Here's how the part is built. I have some questions about the finished solid (model axes, mm). Face numbers are marked on the shaded views. Round coordinates to 2 decimals unless told otherwise and drop trailing zeros. Order: outer loops, then holes, each group sorted by start corner. A loop starts at its lowest first (then second) coordinate and runs counter-clockwise, first axis right, second up. Notation, with made-up numbers: M -20,53.25 L -15,53.25 A10 ccw -15,62.25 Z; hole C 38.25,-33.5 d7. An arc over 180 degrees is marked long. Write item = value, one per line. Start each with the question number.
Item 1: I want a section at B-B, the plane x = 45.5. List the corners of the cut face in (y, z) for me.
Item 2: I want a section at D-D, the plane x = -44. List the corners of the cut face in (y, z) for me, plus the area to 3 significant figures.
Item 3: I want a section at C-C, the plane z = 1.5. List the corners of the cut face in (x, y) for me, plus the area to 3 significant figures.
Item 4: Please list where these lines run through material, in increasing order: L1, parallel to Z at x = 26.5, y = 3.75; L2, parallel to X at y = 3.5, z = -37.5; L3, parallel to X at y = 7, z = 4.
Item 5: We'd pull the mould along X, two halves only. Please class the marked faces 1, 2, 3 and 4: pulls with the +X half, pulls with the -X half, needs draft (parallel to the pull), parting line crosses it, or undercut.
Item 6: I want a section at A-A, the plane y = 7. List the corners of the cut face in (x, z) for me, plus the area to 3 significant figures.
Item 7: I'm going to push flat-ended pins straight in: P1, Ø2.5, axis at x = -32.5, y = 6.5, coming from the -Z side; P2, Ø5, axis at x = -43.5, y = 3, coming from the -Z side; P3, Ø2.5, axis at y = 3, z = -47, coming from the +X side; P4, Ø5, axis at y = 8, z = -39.5, coming from the +X side. Where does each tip first touch, or does it pass through?
```python
from build123d import *

# Parameters (mm, degrees)
SKETCH_1_W      = 99
SKETCH_1_H      = 1.099776848
SKETCH_1_W_2    = 4.3
SKETCH_1_H_2    = 20
SKETCH_1_W_3    = 19.968743504
SKETCH_1_H_3    = 0.87958721
EXTRUDE_6_DEPTH = 10
SKETCH_1_15_W   = 99
SKETCH_1_15_H   = 18.900223152
EXTRUDE_7_DEPTH = 5


with BuildPart() as part:
    # Sketch 1 → Extrude 6 (new body)
    with BuildSketch(Plane(origin=(0, 0, 0), x_dir=(1, 0, 0), z_dir=(0, 1, 0))):
        Polygon((-63.8, 10), (-63.8, -10), (-59.5, -10), (-59.5, -8.900223152), (-59.5, 10), align=None)
        with Locations((-10, -9.450111576)):
            Rectangle(SKETCH_1_W, SKETCH_1_H)
        with Locations((61.65, 0)):
            Rectangle(SKETCH_1_W_2, SKETCH_1_H_2)
        with Locations((49.484371752, 75.060206395)):
            Rectangle(SKETCH_1_W_3, SKETCH_1_H_3)
    extrude(amount=EXTRUDE_6_DEPTH)

    # Sketch 1_15 → Extrude 7 (add)
    with BuildSketch(Plane(origin=(0, 0, 0), x_dir=(1, 0, 0), z_dir=(0, 1, 0))):
        with Locations((-10, 0.549888424)):
            Rectangle(SKETCH_1_15_W, SKETCH_1_15_H)
        Polygon((39.5, -8.900223152), (39.5, -10), (59.5, -10), (59.5, 10), (39.5, 10), align=None)
        Polygon((39.5, 74.62041279), (39.5, 10), (59.5, 10), (59.5, 75.5), (59.468743504, 75.5), (59.468743504, 74.62041279), align=None)
    extrude(amount=EXTRUDE_7_DEPTH)


solid = part.part
```
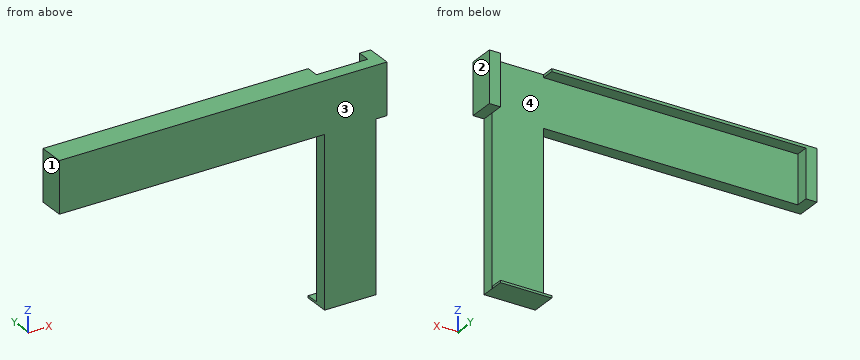
Filled in:
q1.outline = M 0,-75.5 L 10,-75.5 L 10,-74.62 L 5,-74.62 L 5,10 L 0,10 Z
q2.outline = M 0,-10 L 5,-10 L 5,8.9 L 10,8.9 L 10,10 L 0,10 Z
q2.area = 105 mm^2
q3.outline = M -63.8,0 L 63.8,0 L 63.8,10 L 59.5,10 L 59.5,5 L -59.5,5 L -59.5,10 L -63.8,10 Z
q3.area = 681 mm^2
q4.L1 = -10 to 10
q4.L2 = 39.5 to 59.5
q4.L3 = -63.8 to -59.5, 59.5 to 63.8
q5.face_1 = pulls with the -X half
q5.face_2 = pulls with the +X half
q5.face_3 = needs draft
q5.face_4 = undercut
q6.outline = M -63.8,-10 L -59.5,-10 L -59.5,8.9 L 39.5,8.9 L 39.5,10 L -63.8,10 Z; M 39.5,-75.5 L 59.47,-75.5 L 59.47,-74.62 L 39.5,-74.62 Z; M 59.5,-10 L 63.8,-10 L 63.8,10 L 59.5,10 Z
q6.area = 298 mm^2
q7.P1 = 8.9
q7.P2 = -10
q7.P3 = 59.5
q7.P4 = through
